Geometry: final body of the model. Coordinates: model frame, mm. A direction names the side the tool comes from. Give positions to 0.01 mm unless a question says otherwise; leave off trailing zeros. Write each loop counter-clockwise with the first axis right and the second up, starting at its lowest first coordinate (ties: lowest second). Pieces come first, ordered by that corner, then holes. Notation, with made-up numbers: (80.25, 23) -> (91.25, 23) arc R33 ccw to (91.25, 51) -> close; hole circle Ø7 at (-24, -40). An arc over 180 degrees is marked (long way). Answer in a Markdown table with one row per item. Add a question column.
Item 1: Access query for faces 4 (the cylindrical face through (21.983, 4.793, 0.789)), 5 (the flat face through (23, 1, 0)). Directions: +Z, -Z, +X, -X, +Y, -Y. A direction counts if a zero-diameter tool reaches every point of the face in a straight line with its end or side. Return the directions, or none.
Item 2: Section query B-B on x = -3.5. State how many separate pieces and enclosed holes the cut face has, plus the area to 3 significant figures.
Item 3: Draft query along Y for faces 1 (the cylindrical face through (-39.35, -3.92, 0.81)), 2 (the flat face through (-50, 1, 1.599)), 3 (the cylindrical face through (-27.96, 40.35, 0.79)). Return one class per face: +Y half, -Y half, draft (parallel to the pull), parting line (faces both ways), or undercut.
Item 4: Section query D-D on x = -45. Output: boundary loops of the cut face in (y, z).
Item 5: Material intervals for probe 1 along X at (y, z) = (-42.5, 1.25) (3 decimals); probe 2 along X at (y, z) = (26, 0.65); probe 3 along Y at (x, z) = (29.5, 0.9), sorted ascending. Write a range as from..to.
Item 6: First-contact query: P1, Ø0.8, axis at x = -51, z = 1, coming from the -Y side; P2, Ø3, axis at x = -4, y = 37.5, coming from the +Z side; P3, Ø0.5, axis at x = 44, z = 0.5, coming from the -Y side; P4, Ø0.8, axis at y = -44.5, z = 1, coming from the -X side. Flat tips, straight axial feed; report the tip coordinate or a pass-through.
```python
from build123d import *

# Parameters (mm, degrees)
SKETCH1_W                           = 106
SKETCH1_H                           = 106
MAINOUTLINE_DEPTH                   = 1.6
SKETCH4_W                           = 11.7
SKETCH4_H                           = 11.7
RAILCUTOUTS_DEPTH                   = 75.970394157
SKETCH13_W                          = 5.7
SKETCH13_H                          = 1.9
SKETCH13_W_2                        = 1.8
SKETCH13_H_2                        = 3
FILLETCUTOUTS_DEPTH                 = 75.970394157
SMOOTHCORNER_DEPTH                  = 10
MIRROR2_COPY_1_SKETCH_W             = 11.7
MIRROR2_COPY_1_SKETCH_H             = 11.7
MIRROR2_COPY_1_DEPTH                = 75.970394157
MIRROR2_COPY_2_SKETCH_W             = 5.7
MIRROR2_COPY_2_SKETCH_H             = 1.9
MIRROR2_COPY_2_SKETCH_W_2           = 1.8
MIRROR2_COPY_2_SKETCH_H_2           = 3
MIRROR2_COPY_2_DEPTH                = 75.970394157
MIRROR2_COPY_3_DEPTH                = 10
MIRROR2_COPY_4_SKETCH_W             = 11.7
MIRROR2_COPY_4_SKETCH_H             = 11.7
MIRROR2_COPY_4_DEPTH                = 75.970394157
MIRROR2_COPY_5_SKETCH_W             = 5.7
MIRROR2_COPY_5_SKETCH_H             = 1.9
MIRROR2_COPY_5_SKETCH_W_2           = 1.8
MIRROR2_COPY_5_SKETCH_H_2           = 3
MIRROR2_COPY_5_DEPTH                = 75.970394157
FILLET10_R                          = 0.5
M2_CLEARANCE_HOLE1_D                = 2.1
INTERBOARDCONNECTORHOLES_DEPTH      = 75.970394157
INTERBOARDCONNECTORHOLES_DEPTH_BACK = 75.970394157
SKETCH12_R                          = 0.8
SKETCH16_W                          = 90
SKETCH16_H                          = 5.2
SKETCH16_W_2                        = 5.2
SKETCH16_H_2                        = 90
CUT_EXTRUDE6_DEPTH                  = 0.001
CUT_EXTRUDE10_DEPTH                 = 75.970394157
CUT_EXTRUDE10_DEPTH_BACK            = 75.970394157
SKETCH21_R                          = 22.5
SKETCH24_OUTSIDE_W                  = 137.984
SKETCH24_OUTSIDE_H                  = 137.984
SKETCH24_OUTSIDE_W_2                = 105.6
SKETCH24_OUTSIDE_H_2                = 105.6
CUT_EXTRUDE19_DEPTH                 = 75.970394157
FILLET7_R                           = 0.5
F_1_0MM_DOWEL_HOLE1_D               = 3.7
CUT_EXTRUDE23_DEPTH                 = 75.687616109
FILLET14_R                          = 1


with BuildPart() as part:
    # Sketch1 → mainOutline (new body)
    with BuildSketch(Plane.XY):
        Rectangle(SKETCH1_W, SKETCH1_H)
    extrude(amount=MAINOUTLINE_DEPTH)

    # Sketch4 → railCutouts (cut, through all)
    with BuildSketch(Plane(origin=(0, 0, 0), x_dir=(-1, 0, 0), z_dir=(0, 0, -1))):
        with Locations((47.15, 47.15)):
            Rectangle(SKETCH4_W, SKETCH4_H)
    railcutouts = extrude(amount=-RAILCUTOUTS_DEPTH, mode=Mode.SUBTRACT)

    # Sketch13 → filletCutouts (cut, symmetric)
    with BuildSketch(Plane(origin=(0, 0, 0), x_dir=(-1, 0, 0), z_dir=(0, 0, -1))):
        with Locations((50.15, 40.35)):
            Rectangle(SKETCH13_W, SKETCH13_H)
        with Locations((40.4, 51.5)):
            Rectangle(SKETCH13_W_2, SKETCH13_H_2)
    filletcutouts = extrude(amount=FILLETCUTOUTS_DEPTH, both=True, mode=Mode.SUBTRACT)

    # Sketch27 → smoothCorner (cut)
    with BuildSketch(Plane.XY.offset(1.6)):
        with BuildLine():
            Line((-40.928025612, 42.198025612), (-40.928025612, 49.628025612))
            Line((-40.928025612, 49.628025612), (-40.398025612, 49.628025612))
            ThreePointArc((-40.398025612, 49.628025612), (-39.5, 50), (-39.128025612, 50.898025612))
            Line((-39.128025612, 50.898025612), (-39.128025612, 53))
            Line((-39.128025612, 53), (-53, 53))
            Line((-53, 53), (-53, 39.028025612))
            Line((-53, 39.028025612), (-48.198025612, 39.028025612))
            ThreePointArc((-48.198025612, 39.028025612), (-47.3, 39.4), (-46.928025612, 40.298025612))
            Line((-46.928025612, 40.298025612), (-46.928025612, 40.928025612))
            Line((-46.928025612, 40.928025612), (-42.198025612, 40.928025612))
            ThreePointArc((-42.198025612, 40.928025612), (-41.3, 41.3), (-40.928025612, 42.198025612))
        make_face()
    smoothcorner = extrude(amount=-SMOOTHCORNER_DEPTH, mode=Mode.SUBTRACT)

    # Mirror1: railCutouts, filletCutouts, smoothCorner across plane
    add(railcutouts.mirror(Plane(origin=(0, 0, 0), x_dir=(0, 0, 1), z_dir=(1, 0, 0))), mode=Mode.SUBTRACT)
    add(filletcutouts.mirror(Plane(origin=(0, 0, 0), x_dir=(0, 0, 1), z_dir=(1, 0, 0))), mode=Mode.SUBTRACT)
    add(smoothcorner.mirror(Plane(origin=(0, 0, 0), x_dir=(0, 0, 1), z_dir=(1, 0, 0))), mode=Mode.SUBTRACT)

    # Mirror2: smoothCorner across plane
    add(smoothcorner.mirror(Plane.ZX), mode=Mode.SUBTRACT)

    # Mirror2 copy 1 sketch → Mirror2 copy 1 (cut, through all)
    with BuildSketch(Plane(origin=(0, 0, 0), x_dir=(1, 0, 0), z_dir=(0, 0, -1))):
        with Locations((47.15, 47.15)):
            Rectangle(MIRROR2_COPY_1_SKETCH_W, MIRROR2_COPY_1_SKETCH_H)
    extrude(amount=-MIRROR2_COPY_1_DEPTH, mode=Mode.SUBTRACT)

    # Mirror2 copy 2 sketch → Mirror2 copy 2 (cut, symmetric)
    with BuildSketch(Plane(origin=(0, 0, 0), x_dir=(1, 0, 0), z_dir=(0, 0, -1))):
        with Locations((50.15, 40.35)):
            Rectangle(MIRROR2_COPY_2_SKETCH_W, MIRROR2_COPY_2_SKETCH_H)
        with Locations((40.4, 51.5)):
            Rectangle(MIRROR2_COPY_2_SKETCH_W_2, MIRROR2_COPY_2_SKETCH_H_2)
    extrude(amount=MIRROR2_COPY_2_DEPTH, both=True, mode=Mode.SUBTRACT)

    # Mirror2 copy 3 sketch → Mirror2 copy 3 (cut)
    with BuildSketch(Plane(origin=(0, 0, 1.6), x_dir=(-1, 0, 0), z_dir=(0, 0, 1))):
        with BuildLine():
            Line((-40.928025612, 42.198025612), (-40.928025612, 49.628025612))
            Line((-40.928025612, 49.628025612), (-40.398025612, 49.628025612))
            ThreePointArc((-40.398025612, 49.628025612), (-39.5, 50), (-39.128025612, 50.898025612))
            Line((-39.128025612, 50.898025612), (-39.128025612, 53))
            Line((-39.128025612, 53), (-53, 53))
            Line((-53, 53), (-53, 39.028025612))
            Line((-53, 39.028025612), (-48.198025612, 39.028025612))
            ThreePointArc((-48.198025612, 39.028025612), (-47.3, 39.4), (-46.928025612, 40.298025612))
            Line((-46.928025612, 40.298025612), (-46.928025612, 40.928025612))
            Line((-46.928025612, 40.928025612), (-42.198025612, 40.928025612))
            ThreePointArc((-42.198025612, 40.928025612), (-41.3, 41.3), (-40.928025612, 42.198025612))
        make_face()
    extrude(amount=-MIRROR2_COPY_3_DEPTH, mode=Mode.SUBTRACT)

    # Mirror2 copy 4 sketch → Mirror2 copy 4 (cut, through all)
    with BuildSketch(Plane(origin=(0, 0, 0), x_dir=(-1, 0, 0), z_dir=(0, 0, -1))):
        with Locations((47.15, -47.15)):
            Rectangle(MIRROR2_COPY_4_SKETCH_W, MIRROR2_COPY_4_SKETCH_H)
    extrude(amount=-MIRROR2_COPY_4_DEPTH, mode=Mode.SUBTRACT)

    # Mirror2 copy 5 sketch → Mirror2 copy 5 (cut, symmetric)
    with BuildSketch(Plane(origin=(0, 0, 0), x_dir=(-1, 0, 0), z_dir=(0, 0, -1))):
        with Locations((50.15, -40.35)):
            Rectangle(MIRROR2_COPY_5_SKETCH_W, MIRROR2_COPY_5_SKETCH_H)
        with Locations((40.4, -51.5)):
            Rectangle(MIRROR2_COPY_5_SKETCH_W_2, MIRROR2_COPY_5_SKETCH_H_2)
    extrude(amount=MIRROR2_COPY_5_DEPTH, both=True, mode=Mode.SUBTRACT)

    # Fillet10
    fillet10_edges = [part.edges().sort_by_distance(p)[0] for p in [
        (40.928025612, 49.628025612, 0.8),
        (46.928025612, 40.928025612, 0.8),
        (46.928025612, -40.928025612, 0.8),
        (40.928025612, -49.628025612, 0.8),
        (-40.928025612, -49.628025612, 0.8),
        (-46.928025612, -40.928025612, 0.8),
        (-46.928025612, 40.928025612, 0.8),
        (-40.928025612, 49.628025612, 0.8),
    ]]
    fillet(fillet10_edges, radius=FILLET10_R)

    # M2 Clearance Hole1 (through all)
    with Locations(Plane(origin=(0, 0, 0), x_dir=(-1, 0, 0), z_dir=(0, 0, -1))):
        with Locations((49.5, -27.5), (27.5, -49.5), (-49.5, -27.5), (-27.5, -49.5), (-27.5, 49.5), (-49.5, 27.5), (27.5, 49.5), (49.5, 27.5)):
            Hole(M2_CLEARANCE_HOLE1_D / 2)

    # Sketch12 → interboardConnectorHoles (cut, two sides: drawn at the far end of the back side and taken through both)
    with BuildSketch(Plane.XY.offset(1.6).offset(-INTERBOARDCONNECTORHOLES_DEPTH_BACK)):
        with Locations((-34.285, -42.5)):
            Circle(SKETCH12_R)
        with Locations((-23.515, -42.5)):
            Circle(SKETCH12_R)
    extrude(amount=INTERBOARDCONNECTORHOLES_DEPTH + INTERBOARDCONNECTORHOLES_DEPTH_BACK, mode=Mode.SUBTRACT)

    # Sketch16 → Cut-Extrude6 (cut)
    with BuildSketch(Plane.XY.offset(1.6)):
        with Locations((0, -50.4)):
            Rectangle(SKETCH16_W, SKETCH16_H)
        with Locations((0, 50.4)):
            Rectangle(SKETCH16_W, SKETCH16_H)
        with Locations((-50.4, 0)):
            Rectangle(SKETCH16_W_2, SKETCH16_H_2)
        with Locations((50.4, 0)):
            Rectangle(SKETCH16_W_2, SKETCH16_H_2)
    extrude(amount=-CUT_EXTRUDE6_DEPTH, mode=Mode.SUBTRACT)

    # Sketch21 → Cut-Extrude10 (cut, two sides: drawn at the far end of the back side and taken through both)
    with BuildSketch(Plane.XY.offset(-CUT_EXTRUDE10_DEPTH_BACK)):
        Circle(SKETCH21_R)
    extrude(amount=CUT_EXTRUDE10_DEPTH + CUT_EXTRUDE10_DEPTH_BACK, mode=Mode.SUBTRACT)

    # Sketch24 outside → Cut-Extrude19 (cut, through all)
    with BuildSketch(Plane.XY.offset(1.6)):
        Rectangle(SKETCH24_OUTSIDE_W, SKETCH24_OUTSIDE_H)
        Rectangle(SKETCH24_OUTSIDE_W_2, SKETCH24_OUTSIDE_H_2, mode=Mode.SUBTRACT)
    extrude(amount=-CUT_EXTRUDE19_DEPTH, mode=Mode.SUBTRACT)

    # Fillet7
    fillet7_edges = [part.edges().sort_by_distance(p)[0] for p in [
        (-52.8, -39.028025612, 0.7995),
        (-39.128025612, -52.8, 0.7995),
        (52.8, -39.028025612, 0.7995),
        (39.128025612, 52.8, 0.7995),
        (52.8, 39.028025612, 0.7995),
        (39.128025612, -52.8, 0.7995),
        (-52.8, 39.028025612, 0.7995),
        (-39.128025612, 52.8, 0.7995),
    ]]
    fillet(fillet7_edges, radius=FILLET7_R)

    # 1.0mm Dowel Hole1 (through all)
    with Locations(Plane(origin=(-37.5, 4, 0), x_dir=(-1, 0, 0), z_dir=(0, 0, -1))):
        with Locations((0, 0), (0, -8), (-33.5, -41.5), (-41.5, -41.5), (-75, -8), (-75, 0), (-41.5, 33.5), (-33.5, 33.5)):
            Hole(F_1_0MM_DOWEL_HOLE1_D / 2)

    # Sketch33 → Cut-Extrude23 (cut, through all)
    with BuildSketch(Plane(origin=(0, 0, 0), x_dir=(-1, 0, 0), z_dir=(0, 0, -1))):
        with BuildLine():
            Line((-7.8, 16.8), (-7.8, 38.8))
            Line((-7.8, 38.8), (-37.8, 38.8))
            ThreePointArc((-37.8, 38.8), (-40.350055679, 27.8), (-37.8, 16.8))
            Line((-37.8, 16.8), (-7.8, 16.8))
        make_face()
        with BuildLine():
            Line((-16.8, -7.8), (-38.8, -7.8))
            Line((-38.8, -7.8), (-38.8, -37.8))
            ThreePointArc((-38.8, -37.8), (-27.8, -40.350055679), (-16.8, -37.8))
            Line((-16.8, -37.8), (-16.8, -7.8))
        make_face()
        with BuildLine():
            Line((16.8, 7.8), (38.8, 7.8))
            Line((38.8, 7.8), (38.8, 37.8))
            ThreePointArc((38.8, 37.8), (27.8, 40.350055679), (16.8, 37.8))
            Line((16.8, 37.8), (16.8, 7.8))
        make_face()
        with BuildLine():
            Line((7.8, -16.8), (7.8, -38.8))
            Line((7.8, -38.8), (37.8, -38.8))
            ThreePointArc((37.8, -38.8), (40.350055679, -27.8), (37.8, -16.8))
            Line((37.8, -16.8), (7.8, -16.8))
        make_face()
    extrude(amount=-CUT_EXTRUDE23_DEPTH, mode=Mode.SUBTRACT)

    # Fillet14
    fillet14_edges = [part.edges().sort_by_distance(p)[0] for p in [
        (14.96696362, 16.8, 0.8),
        (7.8, 21.104738804, 0.8),
        (-16.8, 14.96696362, 0.8),
        (-21.104738804, 7.8, 0.8),
        (-14.96696362, -16.8, 0.8),
        (-7.8, -21.104738804, 0.8),
        (16.8, -14.96696362, 0.8),
        (21.104738804, -7.8, 0.8),
    ]]
    fillet(fillet14_edges, radius=FILLET14_R)


solid = part.part
```
Findings below:
| question | item | result |
|---|---|---|
| 1 | face 4 | +Z, -Z |
| 1 | face 5 | -Z, +X, -X, +Y, -Y |
| 2 | separate pieces | 4 |
| 2 | enclosed holes | 0 |
| 2 | area | 86.4 mm^2 |
| 3 | face 1 | undercut |
| 3 | face 2 | draft |
| 3 | face 3 | undercut |
| 4 | outline | (-40.93, 0) -> (40.93, 0) -> (40.93, 1.6) -> (-40.93, 1.6) -> close |
| 5 | probe 1 | x = -40.928..-35.085, -33.485..-24.315, -22.715..40.928 |
| 5 | probe 2 | x = -52.8..-38.8, -16.8..7.8, 40.29..52.8 |
| 5 | probe 3 | y = -52.8..-40.29, -7.8..16.8, 38.8..52.8 |
| 6 | P1 | stops at y = -39.03 |
| 6 | P2 | passes through |
| 6 | P3 | stops at y = -40.93 |
| 6 | P4 | stops at x = -40.93 |
